Verification items for the finished model (mm, model axes). A direction names the side the tool comes from. Round coordinates to 2 decimals unless told otherwise and drop trailing zeros. Loops run counter-clockwise (first coordinate to the right, second up) from the corner with the lowest first, then second, coordinate; pieces in that order, holes last. Notation, with made-up numbers: M -1.5,43.5 L 11.5,43.5 A34 ccw 11.5,74.5 Z; hole C 69,11 d11. An arc over 180 degrees is marked long. Answer as CSV lines item,"result".
```python
from build123d import *

# Parameters (mm, degrees)
EXTRUDE001_DEPTH = 5
EXTRUDE_DEPTH    = 16


with BuildPart() as cap_top_extrude:
    # Sketch006 → Extrude001 (new body)
    with BuildSketch(Plane.XY):
        with BuildLine():
            ThreePointArc((-7, -12), (0, -19), (7, -12))
            Line((7, -12), (7, 12))
            ThreePointArc((7, 12), (0, 19), (-7, 12))
            Line((-7, -12), (-7, 12))
        make_face()
    extrude(amount=EXTRUDE001_DEPTH)


with BuildPart() as cap_top_extrude_1:
    # Extrude001 placement: moved
    add(cap_top_extrude.part.moved(Location((0, 0, 16))))


with BuildPart() as cap_fuse:
    # Sketch005 → Extrude (new body)
    with BuildSketch(Plane.XY):
        with BuildLine():
            ThreePointArc((-4, -9), (0, -13), (4, -9))
            Line((4, -9), (4, 9))
            ThreePointArc((4, 9), (0, 13), (-4, 9))
            Line((-4, -9), (-4, 9))
        make_face()
    extrude(amount=EXTRUDE_DEPTH)

    # Fusion: union cap_top_extrude
    add(cap_top_extrude_1.part)


solid = cap_fuse.part
```
1) Section check C-C (z = 5.75). Record the cut outline in (x, y).
Here are the results:
outline,"M -4,-9 A4 ccw 4,-9 L 4,9 A4 ccw -4,9 Z"
2) Section check A-A (y = 5). Record the cut outline in (x, z).
Here are the results:
outline,"M -7,16 L -4,16 L -4,0 L 4,0 L 4,16 L 7,16 L 7,21 L -7,21 Z"
3) Set-up check for faces 1 (the cylindrical face through (0, -13, 8)), 2 (the flat face through (4, 0, 8)), 3 (the flat face through (-4, 0, 8)), 4 (the flat face through (5, 0, 16)), 5 (the cylindrical face through (0, 13, 8)): record each of +Z, -Z, +X, -X, +Y, -Y from which the full face is reachable in a straight line by a thin tool's end or side.
Here are the results:
face 1,"-Z, -Y"
face 2,"-Z, +X, +Y, -Y"
face 3,"-Z, -X, +Y, -Y"
face 4,"-Z"
face 5,"-Z, +Y"
4) Section check B-B (x = -2.5). Record the cut outline in (y, z).
Here are the results:
outline,"M -18.54,16 L -12.12,16 L -12.12,0 L 12.12,0 L 12.12,16 L 18.54,16 L 18.54,21 L -18.54,21 Z"
5) Material ranges on probe 1 along Z at (x, y) = (0.5, -17); probe 2 along Y at (x, z) = (-0.25, 3.75); probe 3 along X at (y, z) = (4.5, 3.5), recorded low to high.
Here are the results:
probe 1,"z = 16 to 21"
probe 2,"y = -12.99 to 12.99"
probe 3,"x = -4 to 4"
6) Go/stop test with flat-tipped pins: pin 1 (1 mm diameter, centred on x = 4, z = 17.5, fed in from -Y); pin 2 (1 mm diameter, centred on y = 9.5, z = 5.5, fed in from +X); pin 3 (1.5 mm diameter, centred on y = 11.5, z = 11, fed in from -X). Record where each tip stops, or that it passes through.
Here are the results:
pin 1,"stops at y = -18.06"
pin 2,"stops at x = 4"
pin 3,"stops at x = -3.6"
7) Section check D-D (z = 19). Record the cut outline in (x, y).
Here are the results:
outline,"M -7,-12 A7 ccw 7,-12 L 7,12 A7 ccw -7,12 Z"
